from build123d import *

# Parameters (mm, degrees)
SKETCH1_R                   = 1.5
BOSS_EXTRUDE1_DEPTH         = 6
FILLET1_R                   = 2
TAP_DRILL_FOR_M3_TAP1_D     = 2.5
TAP_DRILL_FOR_M3_TAP1_DEPTH = 10
TAP_DRILL_FOR_M3_TAP1_TIP   = 0.751075774


with BuildPart() as part:
    # Sketch1 → Boss-Extrude1 (new body)
    with BuildSketch(Plane(origin=(0, 0, 0), x_dir=(0, 0, -1), z_dir=(1, 0, 0))):
        with BuildLine():
            Line((0, 0), (0, 5))
            ThreePointArc((0, 5), (30.306872644, 23.131839172), (63.330515184, 35.650191885))
            ThreePointArc((63.330515184, 35.650191885), (64.588559877, 36.701940492), (64.63724154, 38.340989509))
            ThreePointArc((64.63724154, 38.340989509), (59.61305605, 43.365174999), (52.507784789, 43.365174999))
            Line((52.507784789, 43.365174999), (37.965814359, 78.472597235))
            Line((37.965814359, 78.472597235), (66.606079867, 90.335783638))
            ThreePointArc((66.606079867, 90.335783638), (95.908082664, 95.371985071), (124.52441978, 87.305018919))
            ThreePointArc((124.52441978, 87.305018919), (128.697334576, 79.855822577), (123.769732571, 72.882840251))
            Line((123.769732571, 72.882840251), (107.796810512, 66.266639304))
            ThreePointArc((107.796810512, 66.266639304), (108.591313984, 62.851470364), (108.967839824, 59.365377574))
            ThreePointArc((108.967839824, 59.365377574), (123.962972186, 58.5009858), (138.393920133, 54.335783638))
            Line((138.393920133, 54.335783638), (167.034185641, 42.472597235))
            Line((167.034185641, 42.472597235), (152.492215211, 7.365174999))
            ThreePointArc((152.492215211, 7.365174999), (145.029217261, 7.208101321), (140.094434117, 1.607304426))
            ThreePointArc((140.094434117, 1.607304426), (140.023749539, 1.307301346), (140, 1))
            Line((140, 1), (140, 0))
            Line((140, 0), (120, 0))
            Line((120, 0), (120, 1))
            ThreePointArc((120, 1), (119.627466942, 2.162476387), (118.648648649, 2.891891892))
            ThreePointArc((118.648648649, 2.891891892), (70, 11), (21.351351351, 2.891891892))
            ThreePointArc((21.351351351, 2.891891892), (20.372533058, 2.162476387), (20, 1))
            Line((20, 1), (20, 0))
            Line((20, 0), (0, 0))
        make_face()
        with Locations((80, 58)):
            Circle(SKETCH1_R, mode=Mode.SUBTRACT)
        with Locations((125, 22)):
            Circle(SKETCH1_R, mode=Mode.SUBTRACT)
        with BuildLine():
            Line((105.500709917, 71.809916499), (121.473631977, 78.426117447))
            ThreePointArc((121.473631977, 78.426117447), (122.705532478, 80.169363028), (121.662303779, 82.031662113))
            ThreePointArc((121.662303779, 82.031662113), (95.594542214, 89.380182973), (68.902180461, 84.792506443))
            Line((68.902180461, 84.792506443), (45.805192149, 75.225420634))
            Line((45.805192149, 75.225420634), (55.75496139, 51.204552788))
            Line((55.75496139, 51.204552788), (98.054425187, 68.725564374))
            ThreePointArc((98.054425187, 68.725564374), (97.126892249, 70.151936549), (96.086933305, 71.498539803))
            ThreePointArc((96.086933305, 71.498539803), (96.579960639, 77.133868015), (102.21528885, 76.640840681))
            ThreePointArc((102.21528885, 76.640840681), (103.979962296, 74.308323282), (105.500709917, 71.809916499))
        make_face(mode=Mode.SUBTRACT)
        with BuildLine():
            Line((63.72452745, 48.011301935), (100.350525782, 63.182287179))
            ThreePointArc((100.350525782, 63.182287179), (100.807496311, 60.83691686), (100.995074214, 58.454817254))
            ThreePointArc((100.995074214, 58.454817254), (90.445167867, 55.712658084), (80.47558022, 51.305018919))
            ThreePointArc((80.47558022, 51.305018919), (76.302665424, 43.855822577), (81.230267429, 36.882840251))
            Line((81.230267429, 36.882840251), (97.203189488, 30.266639304))
            ThreePointArc((97.203189488, 30.266639304), (96.003949868, 22.478619602), (96.9455023, 14.655263189))
            ThreePointArc((96.9455023, 14.655263189), (53.555187376, 16.130809763), (11.438572835, 5.591006803))
            ThreePointArc((11.438572835, 5.591006803), (37.27128416, 19.770562369), (64.953613309, 29.873899607))
            ThreePointArc((64.953613309, 29.873899607), (69.985792082, 34.080894036), (70.180518735, 40.637090103))
            ThreePointArc((70.180518735, 40.637090103), (67.559666076, 44.855738901), (63.72452745, 48.011301935))
        make_face(mode=Mode.SUBTRACT)
        with BuildLine():
            Line((106.945574813, 32.725564374), (149.24503861, 15.204552788))
            Line((149.24503861, 15.204552788), (159.194807851, 39.225420634))
            Line((159.194807851, 39.225420634), (136.097819539, 48.792506443))
            ThreePointArc((136.097819539, 48.792506443), (109.405457786, 53.380182973), (83.337696221, 46.031662113))
            ThreePointArc((83.337696221, 46.031662113), (82.294467522, 44.169363028), (83.526368023, 42.426117447))
            Line((83.526368023, 42.426117447), (99.499290083, 35.809916499))
            ThreePointArc((99.499290083, 35.809916499), (101.020037704, 38.308323282), (102.78471115, 40.640840681))
            ThreePointArc((102.78471115, 40.640840681), (108.420039361, 41.133868015), (108.913066695, 35.498539803))
            ThreePointArc((108.913066695, 35.498539803), (107.873107751, 34.151936549), (106.945574813, 32.725564374))
        make_face(mode=Mode.SUBTRACT)
        with BuildLine():
            Line((104.649474218, 27.182287179), (141.27547255, 12.011301935))
            ThreePointArc((141.27547255, 12.011301935), (137.950950961, 9.410732752), (135.464526627, 6))
            Line((135.464526627, 6), (127.541289523, 6))
            ThreePointArc((127.541289523, 6), (116.964502802, 9.762681734), (106.144506127, 12.754982379))
            ThreePointArc((106.144506127, 12.754982379), (104.111850842, 19.835461998), (104.649474218, 27.182287179))
        make_face(mode=Mode.SUBTRACT)
        with BuildLine():
            ThreePointArc((106.5, 58), (104.901854451, 67.063533798), (100.300177743, 75.033871657))
            ThreePointArc((100.300177743, 75.033871657), (98.186929663, 75.218756907), (98.002044413, 73.105508828))
            ThreePointArc((98.002044413, 73.105508828), (102.082776588, 66.037473368), (103.5, 58))
            ThreePointArc((103.5, 58), (105, 56.5), (106.5, 58))
        make_face(mode=Mode.SUBTRACT)
        with BuildLine():
            ThreePointArc((104.699822257, 39.033871657), (100.098145549, 31.063533798), (98.5, 22))
            ThreePointArc((98.5, 22), (100, 20.5), (101.5, 22))
            ThreePointArc((101.5, 22), (102.917223412, 30.037473368), (106.997955587, 37.105508828))
            ThreePointArc((106.997955587, 37.105508828), (106.813070337, 39.218756907), (104.699822257, 39.033871657))
        make_face(mode=Mode.SUBTRACT)
    extrude(amount=BOSS_EXTRUDE1_DEPTH)

    # Fillet1
    fillet1_edges = [part.edges().sort_by_distance(p)[0] for p in [
        (3, 75.225420634, -45.805192149),
        (3, 51.204552788, -55.75496139),
        (3, 68.725564374, -98.054425187),
        (3, 58.454817254, -100.995074214),
        (3, 63.182287179, -100.350525782),
        (3, 48.011301935, -63.72452745),
        (3, 5.591006803, -11.438572835),
        (3, 14.655263189, -96.9455023),
        (3, 30.266639304, -97.203189488),
        (3, 27.182287179, -104.649474218),
        (3, 12.754982379, -106.144506127),
        (3, 6, -127.541289523),
        (3, 6, -135.464526627),
        (3, 12.011301935, -141.27547255),
        (3, 5, 0),
        (3, 43.365174999, -52.507784789),
        (3, 78.472597235, -37.965814359),
        (3, 66.266639304, -107.796810512),
        (3, 59.365377574, -108.967839824),
        (3, 42.472597235, -167.034185641),
        (3, 7.365174999, -152.492215211),
        (3, 39.225420634, -159.194807851),
    ]]
    fillet(fillet1_edges, radius=FILLET1_R)

    # Tap Drill for M3 Tap1
    with Locations(Plane(origin=(0, 0, 0), x_dir=(-1, 0, 0), z_dir=(0, -1, 0))):
        with Locations((-3, 10), (-3, 130)):
            Hole(TAP_DRILL_FOR_M3_TAP1_D / 2, depth=TAP_DRILL_FOR_M3_TAP1_DEPTH)
            with Locations((0, 0, -(TAP_DRILL_FOR_M3_TAP1_DEPTH + TAP_DRILL_FOR_M3_TAP1_TIP / 2))):  # 118° drill point
                Cone(0, TAP_DRILL_FOR_M3_TAP1_D / 2, TAP_DRILL_FOR_M3_TAP1_TIP, mode=Mode.SUBTRACT)


solid = part.part
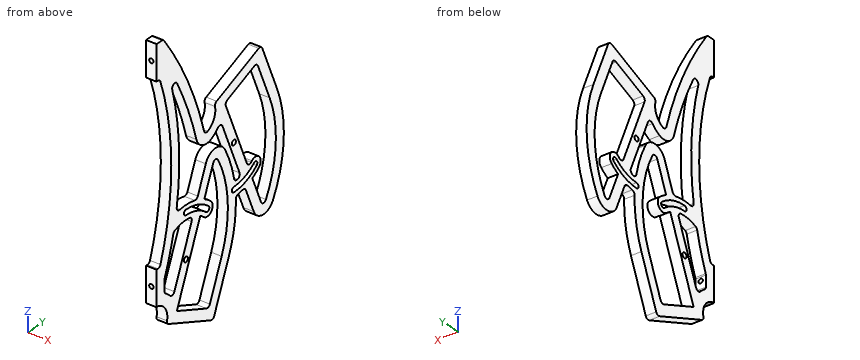
Geometry check sheet. Reference: the model listing, model coordinates, mm. Give positions to 0.01 mm unless a question says otherwise; leave off trailing zeros. Write each loop counter-clockwise with the first axis right and the second up, starting at its lowest first coordinate (ties: lowest second). Pieces come first, ordered by that corner, then holes.
1) Cross-section at B-B (z = -60.5). Record the boundary of the cut face in (x, y), plus the area to 3 significant figures.
Values follow:
outline: (0, 10.7) - (6, 10.7) - (6, 16.71) - (0, 16.71) - close; (0, 28.56) - (6, 28.56) - (6, 34.83) - (0, 34.83) - close; (0, 42.94) - (6, 42.94) - (6, 53.17) - (0, 53.17) - close; (0, 81.31) - (6, 81.31) - (6, 87.81) - (0, 87.81) - close
area: 174 mm2
2) Thickness scan on line 1 (Z direction, x = 4, y = 63); line 2 (Y direction, x = 1.75, z = -137); line 3 (X direction, y = 3, z = -10). Record the ranges inside material, lowest first.
Values follow:
line 1: z = -108.57 to -106.02, -102.96 to -84.23, -50.87 to -44.37
line 2: y = 0 to 8.33, 13.78 to 20.28, 48.42 to 54.9
line 3: x = 0 to 1.75, 4.25 to 6
3) Cross-section at A-A (z = -36). Record the boundary of the cut face in (x, y).
Values follow:
outline: (0, 7.1) - (6, 7.1) - (6, 13.25) - (0, 13.25) - close; (0, 19.19) - (6, 19.19) - (6, 25.78) - (0, 25.78) - close
4) Go/stop test with flat-tipped pins: pin 1 Ø2 at (x, z) = (3, -130) entering from -Y; pin 2 Ø2 at (x, z) = (3, -10) entering from +Y; pin 3 Ø2 at (x, y) = (4.5, 28.5) entering from +Z. Record where each tip stops, or that it passes through.
Values follow:
pin 1: stops at y = 16.27
pin 2: stops at y = 12.43
pin 3: stops at z = -39.98
